```python
from build123d import *

# Parameters (mm, degrees)
SKETCH_2_R          = 9
CUT_EXTRUDE_1_DEPTH = 267.178511668


with BuildPart() as part:
    # Эскиз1 → Повернуть1 (revolve)
    with BuildSketch(Plane.XY, mode=Mode.PRIVATE) as revolve_1_sk:
        with BuildLine():
            Line((-125, 0), (-125, 53))
            Line((-125, 53), (-151.5, 53))
            Line((-151.5, 53), (-151.5, 49))
            Line((-151.5, 49), (-185, 49))
            Line((-185, 49), (-185, 33))
            ThreePointArc((-185, 33), (-184.414213562, 31.585786438), (-183, 31))
            Line((-183, 31), (-149.961434147, 31))
            ThreePointArc((-149.961434147, 31), (-145.422843479, 29.329277132), (-143.050746302, 25.114627072))
            Line((-143.050746302, 25.114627072), (-139, 0))
            Line((-139, 0), (-125, 0))
        make_face()
    revolve(revolve_1_sk.sketch.rotate(Axis((0, 0, 0), (0, 1, 0)), 270), axis=Axis((0, 0, 0), (0, 1, 0)))

    # Эскиз2 → Вырез-Вытянуть1 (cut, through all)
    with BuildSketch(Plane(origin=(0, 49, 0), x_dir=(1, 0, 0), z_dir=(0, 1, 0))):
        with Locations(Location((-167.5, 0, 0), (0, 0, 270))):
            Circle(SKETCH_2_R)
        with Locations(Location((-145.059255134, 83.75, 0), (0, 0, 270))):
            Circle(SKETCH_2_R)
        with Locations(Location((-83.75, 145.059255134, 0), (0, 0, 270))):
            Circle(SKETCH_2_R)
        with Locations(Location((0, 167.5, 0), (0, 0, 270))):
            Circle(SKETCH_2_R)
        with Locations(Location((83.75, 145.059255134, 0), (0, 0, 270))):
            Circle(SKETCH_2_R)
        with Locations(Location((145.059255134, 83.75, 0), (0, 0, 270))):
            Circle(SKETCH_2_R)
        with Locations(Location((167.5, 0, 0), (0, 0, 270))):
            Circle(SKETCH_2_R)
        with Locations(Location((145.059255134, -83.75, 0), (0, 0, 270))):
            Circle(SKETCH_2_R)
        with Locations(Location((83.75, -145.059255134, 0), (0, 0, 270))):
            Circle(SKETCH_2_R)
        with Locations(Location((0, -167.5, 0), (0, 0, 270))):
            Circle(SKETCH_2_R)
        with Locations(Location((-83.75, -145.059255134, 0), (0, 0, 270))):
            Circle(SKETCH_2_R)
        with Locations(Location((-145.059255134, -83.75, 0), (0, 0, 270))):
            Circle(SKETCH_2_R)
    extrude(amount=-CUT_EXTRUDE_1_DEPTH, mode=Mode.SUBTRACT)


solid = part.part
```
Here's how the part is built. I have some questions about the finished solid (model axes, mm). A direction names the side the tool comes from. Coordinates: 2 decimals unless noted, no trailing zeros. Order: outer loops, then holes, each group sorted by start corner. A loop starts at its lowest first (then second) coordinate and runs counter-clockwise, first axis right, second up.
1) Imagine slicing it at A-A on z = 0. List the corners of the cut face in (x, y) for me, and give its area (3 significant figures).
2) We'd pull the mould along Z, two halves only. Please class faces 1 (the face through (152.648, 40.126, -78.912)), 2 (the face through (-152, 49, -1)), 3 (the face through (-41.81, 1.22, -132.77)): +Z half, -Z half, draft (parallel to the pull), parting line (faces both ways), or undercut.
3) Which directions (+Z, -Z, +X, -X, +Y, -Y) give clear straight access to the entire face, cutting with the end or side of a thin tool? Please do faces 4 (the face through (-150, 31, -13)), 5 (the face through (176.423, 40.126, -1.172)), 6 (the face through (-45.506, 50.972, -144.504)).
4) Imagine slicing it at B-B on y = 42.5. State how many separate pieces and enclosed holes the cut face has, and give its area (3 significant figures).
5) Will these pins go through, and if not, where does the flat tip stop? pin 1 (11 mm diameter, centred on x = -83.75, z = 145.06, fed in from -Y); pin 2 (1.5 mm diameter, centred on y = 27.5, z = 23, fed in from +X); pin 3 (3 mm diameter, centred on y = 31.5, z = 33.5, fed in from +X); pin 4 (1 mm diameter, centred on x = -109.5, z = 122, fed in from -Y).
6) I need wall thicknesses on line 1 (X direction, y = 45, z = 0); line 2 (Z direction, x = -83, y = 42); line 3 (X direction, y = 44.75, z = 83.75). Which ranges of each line are inside material? Lowest first, please.
Response values:
1. outline: (-185, 33) arc R2 ccw to (-183, 31) - (-176.5, 31) - (-176.5, 49) - (-185, 49) - close; (-158.5, 31) - (-149.96, 31) arc R7 cw to (-143.05, 25.11) - (-139, 0) - (-125, 0) - (-125, 53) - (-151.5, 53) - (-151.5, 49) - (-158.5, 49) - close; (125, 0) - (139, 0) - (143.05, 25.11) arc R7 cw to (149.96, 31) - (158.5, 31) - (158.5, 49) - (151.5, 49) - (151.5, 53) - (125, 53) - close; (176.5, 31) - (183, 31) arc R2 ccw to (185, 33) - (185, 49) - (176.5, 49) - close
1. area: 2,760 mm2
2. face 1: undercut
2. face 2: draft
2. face 3: parting line
3. face 4: -Y
3. face 5: +Y, -Y
3. face 6: +Y
4. separate pieces: 1
4. enclosed holes: 13
4. area: 55,400 mm2
5. pin 1: passes through
5. pin 2: stops at x = 142.57
5. pin 3: stops at x = 182.09
5. pin 4: stops at y = 31
6. line 1: x = -185 to -176.5, -158.5 to -125, 125 to 158.5, 176.5 to 185
6. line 2: z = -165.34 to -154.03, -136.09 to -93.47, 93.47 to 136.09, 154.03 to 165.34
6. line 3: x = -164.96 to -154.06, -136.06 to -92.8, 92.8 to 136.06, 154.06 to 164.96
